Autodesk Inventor part; units mm, degrees
ref_plane "YZ Plane" through (0, 0, 0) normal (1, 0, 0) x (0, 1, 0)
ref_plane "XZ Plane" through (0, 0, 0) normal (0, 1, 0) x (-1, 0, 0)
ref_plane "XY Plane" through (0, 0, 0) normal (0, 0, 1) x (1, 0, 0)
sketch "Sketch1" plane through (0, 0, 0) normal (0, 1, 0) x (-1, 0, 0)
  line L0 (0, 0) -> (150, 0)
  line L1 (150, 0) -> (150, -80)
  line L2 (150, -80) -> (0, -80)
  line L3 (0, -80) -> (0, 0)
  line L4 (150, -80) -> (0, -80)
  line L5 (0, -80) -> (0, -40)
  line L6 (0, -40) -> (150, -40)
  line L7 (150, -40) -> (150, -80)
  line L8 (150, -40) -> (100.4, -40)
  line L9 (100.4, -40) -> (87.7, -40)
  line L10 (87.7, -40) -> (62.3, -40)
  line L11 (62.3, -40) -> (49.6, -40)
  line L12 (0, 0) -> (10.578, 0)
  line L13 (10.578, 0) -> (10.578, -80)
  line L14 (10.578, -80) -> (0, -80)
  line L15 (0, -80) -> (0, 0)
  line L16 (10.578, 0) -> (10.578, -27)
  line L17 (10.578, -27) -> (10.578, -52)
  line L18 (10.578, -52) -> (10.578, -77)
  line L19 (150, 0) -> (160.578, 0)
  line L20 (160.578, 0) -> (160.578, -80)
  line L21 (160.578, -80) -> (150, -80)
  line L22 (150, -80) -> (150, 0)
  line L23 (160.578, 0) -> (160.578, -27)
  line L24 (160.578, -27) -> (160.578, -52)
  line L25 (160.578, -52) -> (160.578, -77)
  line L26 (0, 0) -> (-10, 0)
  line L27 (-10, 0) -> (-10, -80)
  line L28 (-10, -80) -> (0, -80)
  line L29 (0, -80) -> (0, 0)
  line L30 (150, 0) -> (175, 0)
  line L31 (175, 0) -> (175, -80)
  line L32 (175, -80) -> (150, -80)
  line L33 (150, -80) -> (150, 0)
  dimension "d0" = 150
  dimension "d1" = 80
  dimension "d2" = 40
  dimension "d3" = 49.6
  dimension "d4" = 12.7
  dimension "d5" = 25.4
  dimension "d6" = 12.7
  dimension "d34" = 10.578
  dimension "d35" = 27
  dimension "d36" = 25
  dimension "d37" = 25
  dimension "d46" = 27
  dimension "d47" = 25
  dimension "d48" = 25
  dimension "d49" = 10
  dimension "d50" = 25
  dimension "d51" = 14.422
extrude "Extrusion1" add sketch "Sketch1" along normal blind 24.46
hole "Hole1" at (-49.6, 0, -40) at (-100.4, 0, -40) direction (0, 1, 0) diameter 3.2 depth 4 tip angle 118
hole "Hole2" at (-87.7, 0, -40) at (-62.3, 0, -40) direction (0, 1, 0) diameter 4.917 depth 15 tip angle 118
hole "Hole4" at (-160.578, 0, -27) at (-160.578, 0, -52) at (-10.578, 0, -27) at (-10.578, 0, -52) direction (0, 1, 0) diameter 6.2 end through all counterbore diameter 11 counterbore depth 6
properties part number "CameraAdapter_part3"
Geometry: final body of the model. Coordinates: model frame, mm. A direction names the side the tool comes from. Round coordinates to 2 decimals unless told otherwise and drop trailing zeros. Order: outer loops, then holes, each group sorted by start corner. A loop starts at its lowest first (then second) coordinate and runs counter-clockwise, first axis right, second up. Notation, with made-up numbers: (72, -15.5) -> (120, -15.5) arc R27 ccw to (120, 18.5) -> close; hole circle Ø1 at (28.25, 70). An arc over 180 degrees is marked (long way). Use one line per item in the form item = value. Start each with the question number.
1. Reachability of faces 5 (the face through (-63.038, 7.605, -42.345)), 6 (the face through (-81, 12, 0)) from +Z, -Z, +X, -X, +Y, -Y: full face, straight path, thin tool, end or side. Return the list, or none.
2. Cut plane A-A (z = -27). Return the cut outline in (x, y), then the cut area to 3 significant figures.
3. Draft query along Z for faces 1 (the face through (-81, 12, -80)), 2 (the face through (-81, 0, -39)), 3 (the face through (-8, 6, -29)), 4 (the face through (-89.773, 7.605, -41.322)). Return one class per face: pulls with the +Z half, pulls with the -Z half, needs draft (parallel to the pull), parting line crosses it, or undercut.
4. Pin query (flat end, axial travel): pin 1 Ø12 at (x, y) = (-156, 16) entering from +Z; pin 2 Ø3 at (x, z) = (-62.3, -40) entering from -Y; pin 3 Ø5.5 at (x, z) = (-160.578, -52) entering from -Y; pin 4 Ø5.5 at (x, z) = (-163, -52.5) entering from -Y. Return the tip coordinate at first contact, or that it passes through.
5. Cut plane B-B (y = 1.75). Count the separate pieces of the cut face and the enclosed holes in it, then the cut area to 3 significant figures.
6. Line query: probe 1 along X at (y, z) = (4.85, -52); probe 2 along X at (y, z) = (10.75, -40); probe 3 along Z at (x, y) = (-160.5, 2.5). Output: solid intervals per line, ascending.
Solution:
q1.face_5 = -Y
q1.face_6 = +Z, +X, -X, +Y, -Y
q2.outline = (-175, 0) -> (-166.08, 0) -> (-166.08, 6) -> (-163.68, 6) -> (-163.68, 24.46) -> (-175, 24.46) -> close; (-157.48, 6) -> (-155.08, 6) -> (-155.08, 0) -> (-16.08, 0) -> (-16.08, 6) -> (-13.68, 6) -> (-13.68, 24.46) -> (-157.48, 24.46) -> close; (-7.48, 6) -> (-5.08, 6) -> (-5.08, 0) -> (10, 0) -> (10, 24.46) -> (-7.48, 24.46) -> close
q2.area = 4,160 mm^2
q3.face_1 = pulls with the -Z half
q3.face_2 = needs draft
q3.face_3 = undercut
q3.face_4 = undercut
q4.pin_1 = 0
q4.pin_2 = 15.58
q4.pin_3 = through
q4.pin_4 = 6
q5.separate_pieces = 1
q5.enclosed_holes = 8
q5.area = 14,400 mm^2
q6.probe_1 = -175 to -166.08, -155.08 to -16.08, -5.08 to 10
q6.probe_2 = -175 to -90.16, -85.24 to -64.76, -59.84 to 10
q6.probe_3 = -80 to -57.5, -46.5 to -32.5, -21.5 to 0
